Here's the drawing with two shaded views (mm, measured from the low corner). I have some questions. Round coordinates to 2 decimals unless told otherwise and drop trailing zeros. Write each question's results on one line, items separated by ' | '.
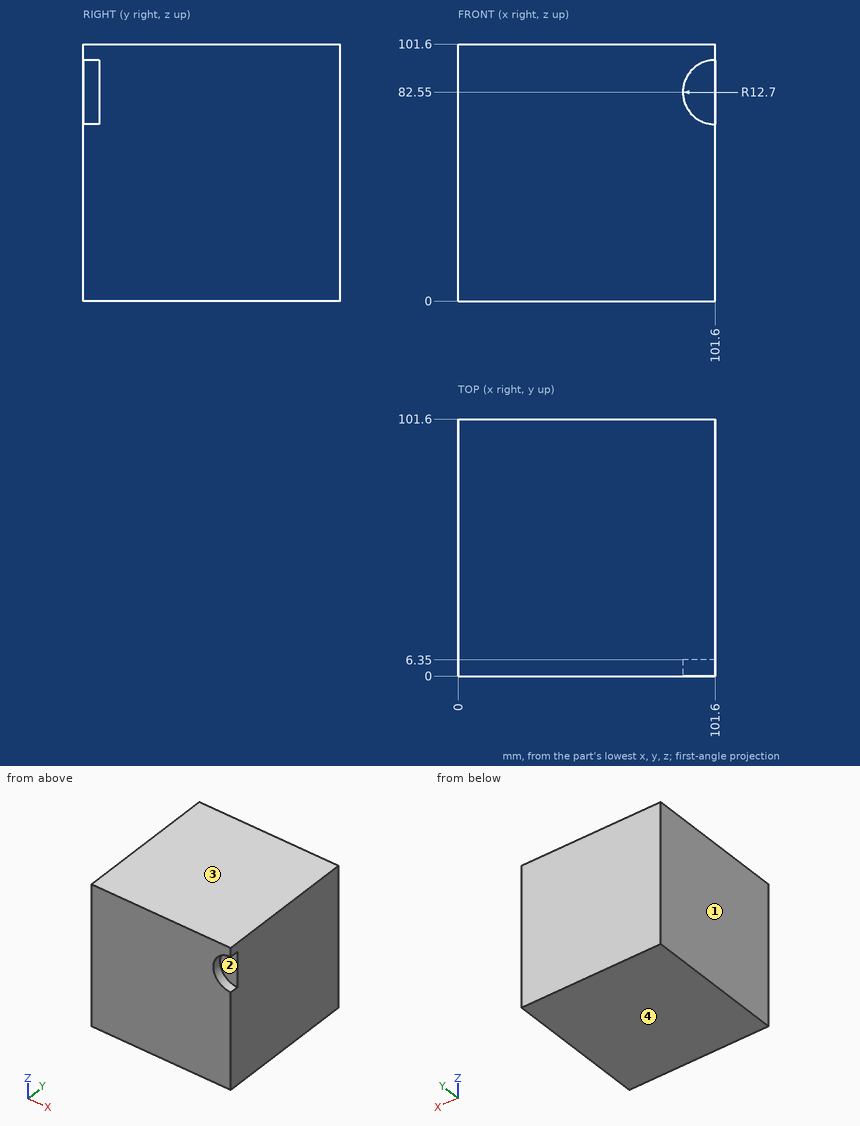
1. We'd pull the mould along Z, two halves only. Please class the marked faces 1, 2, 3 and 4: pulls with the +Z half, pulls with the -Z half, needs draft (parallel to the pull), parting line crosses it, or undercut.
Final values:
face 1: needs draft | face 2: undercut | face 3: pulls with the +Z half | face 4: pulls with the -Z half
2. Will these pins go through, and if not, where does the flat tip stop? pin 1 (6 mm diameter, centred on x = 91, z = 62, fed in from -Y); pin 2 (4 mm diameter, centred on x = 93.5, z = 83, fed in from -Y).
Final values:
pin 1: y = 0 | pin 2: y = 6.35
3. Please list where this line runs through material, in increasing order: line 1 (Y direction, x = 96.5, z = 76). Write a range as from..to.
Final values:
line 1: 6.35..101.6
